from build123d import *

# Parameters (mm, degrees)
SKETCH1_R           = 9.525
BOSS_EXTRUDE1_DEPTH = 1
BOSS_EXTRUDE2_DEPTH = 9.525
SKETCH3_R           = 3.175
CUT_EXTRUDE1_DEPTH  = 18.094644629
SKETCH4_OUTSIDE_W   = 45.884
SKETCH4_OUTSIDE_H   = 45.884
SKETCH4_OUTSIDE_R   = 7.14375
CUT_EXTRUDE2_DEPTH  = 9.525
CUT_EXTRUDE2_DRAFT  = -45


with BuildPart() as part:
    # Sketch1 → Boss-Extrude1 (new body)
    with BuildSketch(Plane.XY):
        Circle(SKETCH1_R)
    extrude(amount=BOSS_EXTRUDE1_DEPTH)

    # Sketch2 → Boss-Extrude2 (add)
    with BuildSketch(Plane.XY.offset(1)):
        Polygon((4.124445986, -7.14375), (8.248891971, 0), (4.124445986, 7.14375), (-4.124445986, 7.14375), (-8.248891971, 0), (-4.124445986, -7.14375), align=None)
    extrude(amount=BOSS_EXTRUDE2_DEPTH)

    # Sketch3 → Cut-Extrude1 (cut, through all)
    with BuildSketch(Plane.XY.offset(10.525)):
        Circle(SKETCH3_R)
    extrude(amount=-CUT_EXTRUDE1_DEPTH, mode=Mode.SUBTRACT)


with BuildPart() as cut_extrude2_tool:
    # Sketch4 outside → Cut-Extrude2 (with draft: the straight prism first)
    with BuildSketch(Plane.XY.offset(10.525)):
        Rectangle(SKETCH4_OUTSIDE_W, SKETCH4_OUTSIDE_H)
        Circle(SKETCH4_OUTSIDE_R, mode=Mode.SUBTRACT)
    extrude(amount=-CUT_EXTRUDE2_DEPTH)
    # Cut-Extrude2: the draft: its side faces are tilted about the plane it starts from
    cut_extrude2_sides = [cut_extrude2_tool.faces().sort_by_distance(p)[0] for p in [
        (0, -22.942, 5.7625),
        (22.942, 0, 5.7625),
        (0, 22.942, 5.7625),
        (-22.942, 0, 5.7625),
        (-7.14375, 0, 5.7625),
    ]]
    draft(cut_extrude2_sides, Plane.XY.offset(10.525), CUT_EXTRUDE2_DRAFT)


with BuildPart() as part_1:
    add(part.part)

    # Cut-Extrude2: cut by cut_extrude2_tool
    add(cut_extrude2_tool.part, mode=Mode.SUBTRACT)


solid = part_1.part
Geometry: final body of the model. Coordinates: model frame, mm. A direction names the side the tool comes from. Give positions to 0.01 mm unless a question says otherwise; leave off trailing zeros. Loops run counter-clockwise (first coordinate to the right, second up) from the corner with the lowest first, then second, coordinate; pieces in that order, holes last. Notation, with made-up numbers: (-15.5, -19.75) -> (35.5, -19.75) arc R23 cw to (35.5, 13.25) -> close; hole circle Ø11 at (26.5, 11). An arc over 180 degrees is marked (long way). Put each result on its own line as item: value.
1. Cut plane A-A (z = 4). Return the cut outline in (x, y) (3 decimals).
Taken from the geometry:
outline: (-8.249, 0) -> (-4.124, -7.144) -> (4.124, -7.144) -> (8.249, 0) -> (4.124, 7.144) -> (-4.124, 7.144) -> close; hole circle Ø6.35 at (0, 0)
2. Ray query, line 1 along Y through (x, z) = (0, 6.5) (3 decimals); line 2 along Z through (x, y) = (1.75, 8.5); line 3 along X through (y, z) = (1.25, 2.75). Return the intervals inside material, ascending. Write a range as [from, to].
Taken from the geometry:
line 1: y = [-7.144, -3.175], [3.175, 7.144]
line 2: z = [0, 1]
line 3: x = [-7.53, -2.92], [2.92, 7.53]
3. Pull-direction query (X, two-part tool) for faces 1 (the conical face through (7.41, -0.02, 10.26)), 2 (the flat face through (1.5, -3.1, 10.525)), 3 (the conical face through (-3.72, -6.41, 10.26)), 4 (the cylindrical face through (-0.69, -3.1, 5.34)); classes: released by +X, released by -X, zero draft, split by the parting line, or undercut.
Taken from the geometry:
face 1: released by +X
face 2: zero draft
face 3: released by -X
face 4: undercut
4. Cut plane B-B (y = 8). Return the cut outline in (x, z).
Taken from the geometry:
outline: (-5.17, 0) -> (5.17, 0) -> (5.17, 1) -> (-5.17, 1) -> close
5. Set-up query: faces 5 (the flat face through (6.216, 3.522, 5.696)), 6 (the flat face through (6, -5, 1)), 7 (the flat face through (6.16, -3.62, 5.7)). Return all of +Z, -Z, +X, -X, +Y, -Y with unobstructed straight access to the full face (end or side cutting, diameter ignored); none if empty.
Taken from the geometry:
face 5: +Z, +X, +Y
face 6: +Z
face 7: +Z, +X, -Y
6. Pin query (flat end, axial travel): P1, Ø3, axis at x = -3.5, z = 8.5, coming from the +Y side; P2, Ø6, axis at x = 3, z = 2, coming from the +Y side; P3, Ø4, axis at x = 0, y = 0, coming from the +Z side; P4, Ø3, axis at y = -1, z = 4.5, coming from the -X side. Return the tip coordinate at first contact, or that it passes through.
Taken from the geometry:
P1: stops at y = 7.14
P2: stops at y = 9.52
P3: passes through
P4: stops at x = -8.25
